For this review, take the finished solid that the model builds, in its own axes (mm). A direction names the side the tool comes from. Give positions to 0.01 mm unless a question says otherwise; leave off trailing zeros. Order: outer loops, then holes, each group sorted by start corner. A loop starts at its lowest first (then second) coordinate and runs counter-clockwise, first axis right, second up. Notation, with made-up numbers: (-11, -26.75) -> (-5, -26.75) arc R11 cw to (-5, -14.75) -> close; hole circle Ø8 at (36.5, 36.5). An arc over 180 degrees is marked (long way). Return JSON: item names as keys, results as strings. Group by question number.
1) For faces 1 (the face through (-1, -15, -19)), 2 (the face through (23, -17, 7)), 3 (the face through (-36.196, -26.111, 0.266)), list the 3-axis set-ups (+Z, -Z, +X, -X, +Y, -Y) from which the entire face can be reached by the end or side of a thin tool; tool diameter is ignored.
2) Add section A-A (z = -11.5). State how many separate pieces and enclosed holes the cut face has, then the cut area to 3 significant figures.
3) Add section C-C (y = -43). Give the boundary of the cut face in (x, z).
4) Insertion check: P1, Ø19, axis at x = 14.5, z = 0, coming from the -Y side; P2, Ø9, axis at x = 15, z = -11.5, coming from the +Y side; P3, Ø5, axis at x = -34.5, z = -14.5, coming from the +Y side. Each pin has a flat end and moves straight along its axis. Give the tip position at first contact, or say it passes through.
5) To check wall thickness, follow line 1 along Z through (x, y) = (15, -5); line 2 along X through (y, z) = (-12, -11); line 3 along X through (y, z) = (1.75, -11.5). State the ranges of each line that lie inside material, in increasing order.
6) Add section B-B (x = -15). Give the boundary of the cut face in (y, z), then the cut area to 3 significant figures.
7) The part is to be moulded in two halves that separate along X. For faces 4 (the face through (-45.6, -47.3, -0.3)), 5 (the face through (-1, -15, 19)), 6 (the face through (16.64, -12.54, -14.07)), say which applies: released by +X, released by -X, zero draft, split by the parting line, or undercut.
8) Add section D-D (x = 23). Give the boundary of the cut face in (y, z).
from build123d import *

# Parameters (mm, degrees)
BOSS_EXTRUDE1_DEPTH = 19
CUT_EXTRUDE8_DEPTH  = 39
FILLET1_R           = 6
SKETCH2_R           = 3.05
CUT_EXTRUDE1_DEPTH  = 42
SKETCH3_R           = 5.5
CUT_EXTRUDE2_DEPTH  = 7
SKETCH8_R           = 2.9
CUT_EXTRUDE7_DEPTH  = 23
CHAMFER2_SIZE       = 5


with BuildPart() as part:
    # Sketch1 → Boss-Extrude1 (new body, symmetric)
    with BuildSketch(Plane.XY):
        Polygon((48.1, 6), (-48.1, 6), (-48.1, -49.8), (-38, -49.8), (-38, -24.4), (38, -24.4), (38, -49.8), (48.1, -49.8), align=None)
    extrude(amount=BOSS_EXTRUDE1_DEPTH, both=True)

    # Sketch9 → Cut-Extrude8 (cut, through all)
    with BuildSketch(Plane.XY.offset(19)):
        Polygon((-30, 6), (-48.1, -14.3), (-48.1, 6), align=None)
        Polygon((48.1, 6), (30, 6), (48.1, -14.3), align=None)
    extrude(amount=-CUT_EXTRUDE8_DEPTH, mode=Mode.SUBTRACT)

    # Fillet1
    fillet1_edges = [part.edges().sort_by_distance(p)[0] for p in [
        (38, -24.4, 0),
        (-38, -24.4, 0),
    ]]
    fillet(fillet1_edges, radius=FILLET1_R)

    # Sketch2 → Cut-Extrude1 (cut)
    with BuildSketch(Plane(origin=(0, 6, 0), x_dir=(1, 0, 0), z_dir=(0, 1, 0))):
        with Locations((-15, 11.5)):
            Circle(SKETCH2_R)
        with Locations((15, 11.5)):
            Circle(SKETCH2_R)
    extrude(amount=-CUT_EXTRUDE1_DEPTH, mode=Mode.SUBTRACT)

    # Sketch3 → Cut-Extrude2 (cut)
    with BuildSketch(Plane(origin=(0, 6, 0), x_dir=(1, 0, 0), z_dir=(0, 1, 0))):
        with Locations((-15, 11.5)):
            Circle(SKETCH3_R)
        with Locations((15, 11.5)):
            Circle(SKETCH3_R)
    extrude(amount=-CUT_EXTRUDE2_DEPTH, mode=Mode.SUBTRACT)

    # Sketch8 → Cut-Extrude7 (cut)
    with BuildSketch(Plane(origin=(0, 6, 0), x_dir=(1, 0, 0), z_dir=(0, 1, 0))):
        with Locations((-23, -7)):
            Circle(SKETCH8_R)
        with Locations((23, -7)):
            Circle(SKETCH8_R)
    extrude(amount=-CUT_EXTRUDE7_DEPTH, mode=Mode.SUBTRACT)

    # Chamfer2
    chamfer2_edges = [part.edges().sort_by_distance(p)[0] for p in [
        (48.1, -49.8, 0),
        (-48.1, -49.8, 0),
    ]]
    chamfer(chamfer2_edges, length=CHAMFER2_SIZE)


solid = part.part
Evaluation:
{
 "1": {"face 1": "-Z, +X, -X, +Y, -Y", "face 2": "+Y", "face 3": "+Z, -Z, -Y"},
 "2": {"separate pieces": "3", "enclosed holes": "0", "area": "2,620 mm^2"},
 "3": {"outline": "(-48.1, -19) -> (-38, -19) -> (-38, 19) -> (-48.1, 19) -> close; (38, -19) -> (48.1, -19) -> (48.1, 19) -> (38, 19) -> close"},
 "4": {"P1": "y = -24.4", "P2": "y = -1", "P3": "y = 3.76"},
 "5": {"line 1": "-19 to -14.55, -8.45 to 19", "line 2": "-46.05 to -18.01, -11.99 to 11.99, 18.01 to 46.05", "line 3": "-33.79 to -20.5, -9.5 to 9.5, 20.5 to 33.79"},
 "6": {"outline": "(-24.4, -19) -> (6, -19) -> (6, -17) -> (-1, -17) -> (-1, -14.55) -> (-24.4, -14.55) -> close; (-24.4, -8.45) -> (-1, -8.45) -> (-1, -6) -> (6, -6) -> (6, 19) -> (-24.4, 19) -> close", "area": "935 mm^2"},
 "7": {"face 4": "released by -X", "face 5": "zero draft", "face 6": "undercut"},
 "8": {"outline": "(-24.4, -19) -> (6, -19) -> (6, 4.1) -> (-17, 4.1) -> (-17, 9.9) -> (6, 9.9) -> (6, 19) -> (-24.4, 19) -> close"}
}
